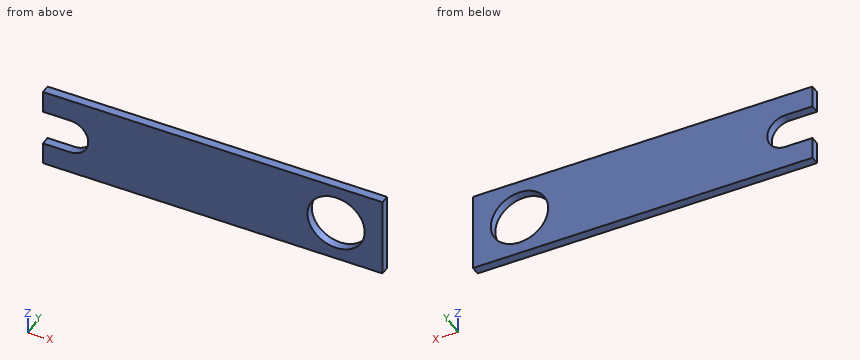
from build123d import *

# Parameters (mm, degrees)
SKETCH1_R           = 21.1
BOSS_EXTRUDE1_DEPTH = 6.35


with BuildPart() as part:
    # Sketch1 → Boss-Extrude1 (new body)
    with BuildSketch(Plane(origin=(0, 0, 0), x_dir=(1, 0, 0), z_dir=(0, 1, 0))):
        with BuildLine():
            Line((-195.75, 13.33), (-215.75, 13.33))
            Line((-215.75, 13.33), (-215.75, 30))
            Line((-215.75, 30), (34.25, 30))
            Line((34.25, 30), (34.25, -30))
            Line((34.25, -30), (-215.75, -30))
            Line((-215.75, -30), (-215.75, -13.33))
            Line((-215.75, -13.33), (-195.75, -13.33))
            ThreePointArc((-195.75, -13.33), (-182.42, 0), (-195.75, 13.33))
        make_face()
        Circle(SKETCH1_R, mode=Mode.SUBTRACT)
    extrude(amount=BOSS_EXTRUDE1_DEPTH)


solid = part.part
Source: CAD feature listing. Evaluate the final solid. Frame: model axes, mm. Give positions to 0.01 mm unless a question says otherwise; leave off trailing zeros. Write each loop counter-clockwise with the first axis right and the second up, starting at its lowest first coordinate (ties: lowest second). Pieces come first, ordered by that corner, then holes. Notation, with made-up numbers: (64, 48) -> (117, 48) arc R29 ccw to (117, 77) -> close; hole circle Ø10 at (26, 87). An arc over 180 degrees is marked (long way). Return JSON: item names as keys, results as strings. Group by question number.
1. Section C-C, the plane x = 0. Output: boundary loops of the cut face in (y, z), then the cut area to 3 significant figures.
2. Section A-A, the plane z = 0. Output: boundary loops of the cut face in (x, y).
3. Material intervals for line 1 (Z direction, x = 0, y = 0.75); line 2 (X direction, y = 2.25, z = 0); line 3 (X direction, y = 0.5, z = -3.5), sorted ascending. Write a range as from..to.
4. Section B-B, the plane y = 3. Output: boundary loops of the cut face in (x, z).
Determined:
{
 "1": {"outline": "(0, -30) -> (6.35, -30) -> (6.35, -21.1) -> (0, -21.1) -> close; (0, 21.1) -> (6.35, 21.1) -> (6.35, 30) -> (0, 30) -> close", "area": "113 mm2"},
 "2": {"outline": "(-182.42, 0) -> (-21.1, 0) -> (-21.1, 6.35) -> (-182.42, 6.35) -> close; (21.1, 0) -> (34.25, 0) -> (34.25, 6.35) -> (21.1, 6.35) -> close"},
 "3": {"line 1": "z = -30..-21.1, 21.1..30", "line 2": "x = -182.42..-21.1, 21.1..34.25", "line 3": "x = -182.89..-20.81, 20.81..34.25"},
 "4": {"outline": "(-215.75, -30) -> (34.25, -30) -> (34.25, 30) -> (-215.75, 30) -> (-215.75, 13.33) -> (-195.75, 13.33) arc R13.33 cw to (-195.75, -13.33) -> (-215.75, -13.33) -> close; hole circle Ø42.2 at (0, 0)"}
}
